Input: part model. Units: mm. Frame: model coordinates. A direction names the side the tool comes from. Give positions to 0.01 mm unless a question says otherwise; leave off trailing zeros. Loops run counter-clockwise (first coordinate to the right, second up) from the corner with the lowest first, then second, coordinate; pieces in that order, holes last. Notation, with made-up numbers: M 61.5,2 L 117.5,2 A21 cw 117.5,25 Z; hole C -6,4 d5. An arc over 180 degrees is marked long. One line per item, written item: value. Start each with the question number.
(1) Section C-C on x = 0. Output: boundary loops of the cut face in (y, z), plus the area to 3 significant figures.
(2) Pull-direction query (X, two-part tool) for faces 3 (the flat face through (-5, -26.5, 2)), 4 (the flat face through (0, 30.5, 2)), 5 (the flat face through (-10, 0, 2)); classes: released by +X, released by -X, zero draft, split by the parting line, or undercut.
(3) Section B-B on z = 2. Output: boundary loops of the cut face in (x, y), plus the area to 3 significant figures.
(4) Ray query, line 1 along Z through (x, y) = (-5, -28.65); line 2 along Y through (x, z) = (0, 3); line 3 along Y through (x, z) = (1.25, 3.35). Return the intervals inside material, ascending. Write a range as from..to.
(5) Pin query (flat end, axial travel): P1, Ø1.2, axis at x = -5, z = 1.5, coming from the -Y side; P2, Ø1.5, axis at x = -6, y = 5.5, coming from the -Z side; P3, Ø6, axis at x = 0, y = 18, coming from the +Z side. Return the tip coordinate at first contact, or that it passes through.
(6) Section A-A on y = 22. Output: boundary loops of the cut face in (x, z).
(7) Access query for faces 1 (the flat face through (10, 0, 2)), 2 (the cylindrical face through (3.8, -28.47, 1.95)). Directions: +Z, -Z, +X, -X, +Y, -Y. A direction counts if a zero-diameter tool reaches every point of the face in a straight line with its end or side. Return the directions, or none.
```python
from build123d import *

# Parameters (mm, degrees)
SCHIZZO1_W                   = 20
SCHIZZO1_H                   = 61
ESTRUSIONE_ESTRUSIONE1_DEPTH = 4
SCHIZZO2_R                   = 5
TAGLIO_ESTRUSIONE1_DEPTH     = 4
FORO_PER_VITE_M2_2_D         = 2.4
FORO_PER_VITE_M2_2_DEPTH     = 4


with BuildPart() as part:
    # Schizzo1 → Estrusione-Estrusione1 (new body)
    with BuildSketch(Plane.XY):
        Rectangle(SCHIZZO1_W, SCHIZZO1_H)
    extrude(amount=ESTRUSIONE_ESTRUSIONE1_DEPTH)

    # Schizzo2 → Taglio-Estrusione1 (cut)
    with BuildSketch(Plane.XY.offset(4)):
        with Locations((0, 18)):
            Circle(SCHIZZO2_R)
    extrude(amount=-TAGLIO_ESTRUSIONE1_DEPTH, mode=Mode.SUBTRACT)

    # Foro per Vite M2-2
    with Locations(Plane(origin=(0, -30.5, 0), x_dir=(-1, 0, 0), z_dir=(0, -1, 0))):
        with Locations((5, -2), (-5, -2)):
            Hole(FORO_PER_VITE_M2_2_D / 2, depth=FORO_PER_VITE_M2_2_DEPTH)


solid = part.part
```
Output values:
1. outline: M -30.5,0 L 13,0 L 13,4 L -30.5,4 Z; M 23,0 L 30.5,0 L 30.5,4 L 23,4 Z
1. area: 204 mm²
2. face 3: undercut
2. face 4: zero draft
2. face 5: released by -X
3. outline: M -10,-30.5 L -6.2,-30.5 L -6.2,-26.5 L -3.8,-26.5 L -3.8,-30.5 L 3.8,-30.5 L 3.8,-26.5 L 6.2,-26.5 L 6.2,-30.5 L 10,-30.5 L 10,30.5 L -10,30.5 Z; hole C 0,18 d10
3. area: 1,120 mm²
4. line 1: z = 0..0.8, 3.2..4
4. line 2: y = -30.5..13, 23..30.5
4. line 3: y = -30.5..13.16, 22.84..30.5
5. P1: stops at y = -26.5
5. P2: stops at z = 0
5. P3: passes through
6. outline: M -10,0 L -3,0 L -3,4 L -10,4 Z; M 3,0 L 10,0 L 10,4 L 3,4 Z
7. face 1: +Z, -Z, +X, +Y, -Y
7. face 2: -Y
